Input: part model. Units: mm. Frame: model coordinates. Face numbers are marked on the shaded views. Coordinates: 2 decimals unless noted, no trailing zeros. Loops run counter-clockwise (first coordinate to the right, second up) from the corner with the lowest first, then second, coordinate; pieces in that order, holes last.
```python
from build123d import *

# Parameters (mm, degrees)
BOSS_EXTRUDE1_DEPTH           = 6.35
F_1_1_4_12_TAPPED_HOLE1_D     = 29.76626
F_1_1_4_12_TAPPED_HOLE1_DEPTH = 74.0791
F_1_1_4_12_TAPPED_HOLE1_TIP   = 8.942686705


with BuildPart() as part:
    # Sketch1 → Boss-Extrude1 (new body)
    with BuildSketch(Plane.XY):
        with BuildLine():
            Line((0, 0), (-25.4, 0))
            Line((-25.4, 0), (-25.4, 6.35))
            Line((-25.4, 6.35), (-18.344682017, 31.55167344))
            ThreePointArc((-18.344682017, 31.55167344), (0, 45.466), (18.344682017, 31.55167344))
            Line((18.344682017, 31.55167344), (25.4, 6.35))
            Line((25.4, 6.35), (25.4, 0))
            Line((25.4, 0), (0, 0))
        make_face()
    extrude(amount=BOSS_EXTRUDE1_DEPTH)

    # 1-1/4-12 Tapped Hole1
    with Locations(Plane(origin=(0, 26.416, 6.35), x_dir=(1, 0, 0), z_dir=(0, 0, 1))):
        with Locations((0, 0)):
            Hole(F_1_1_4_12_TAPPED_HOLE1_D / 2, depth=F_1_1_4_12_TAPPED_HOLE1_DEPTH)
            with Locations((0, 0, -(F_1_1_4_12_TAPPED_HOLE1_DEPTH + F_1_1_4_12_TAPPED_HOLE1_TIP / 2))):  # 118° drill point
                Cone(0, F_1_1_4_12_TAPPED_HOLE1_D / 2, F_1_1_4_12_TAPPED_HOLE1_TIP, mode=Mode.SUBTRACT)


solid = part.part
```
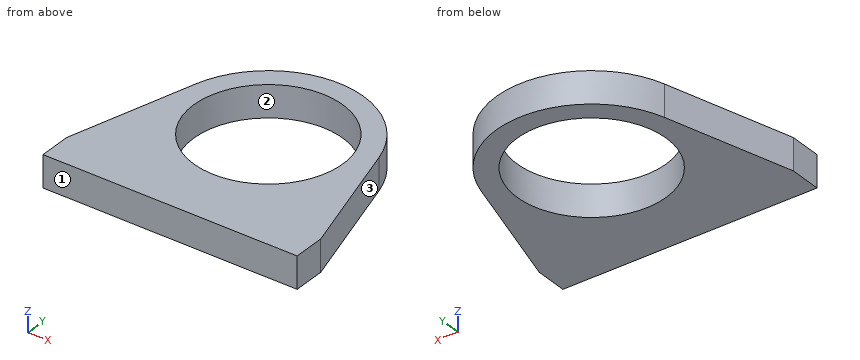
Item 1: Section query D-D (x = 17). Output: boundary loops of the cut face in (y, z).
Result:
outline: (0, 0) - (35.01, 0) - (35.01, 6.35) - (0, 6.35) - close
Item 2: Line query: L1, parallel to Y at x = 0, z = 4.5; L2, parallel to Y at x = -12, z = 1; L3, parallel to X at y = 31, z = 6. Output: solid intervals per line, ascending.
Result:
L1: y = 0 to 11.53, 41.3 to 45.47
L2: y = 0 to 17.61, 35.22 to 41.21
L3: x = -18.5 to -14.16, 14.16 to 18.5
Item 3: Section query A-A (x = 0). Output: boundary loops of the cut face in (y, z).
Result:
outline: (0, 0) - (11.53, 0) - (11.53, 6.35) - (0, 6.35) - close; (41.3, 0) - (45.47, 0) - (45.47, 6.35) - (41.3, 6.35) - close
Item 4: Section query C-C (z = 3). Output: boundary loops of the cut face in (x, y).
Result:
outline: (-25.4, 0) - (25.4, 0) - (25.4, 6.35) - (18.34, 31.55) arc R19.05 ccw to (-18.34, 31.55) - (-25.4, 6.35) - close; hole circle Ø29.77 at (0, 26.42)
Item 5: Section query B-B (y = 38.5). Output: boundary loops of the cut face in (x, z).
Result:
outline: (-14.73, 0) - (-8.69, 0) - (-8.69, 6.35) - (-14.73, 6.35) - close; (8.69, 0) - (14.73, 0) - (14.73, 6.35) - (8.69, 6.35) - close
Item 6: Contact query for flat-ended pins moving along their axis: P1, Ø1, axis at y = 25, z = 5.5, coming from the +X side; P2, Ø6, axis at x = 12.5, y = 4.5, coming from the -Z side; P3, Ø1.5, axis at y = 30.5, z = 2, coming from the -X side. Output: stop coordinate, or through.
Result:
P1: stops at x = 20.32
P2: stops at z = 0
P3: stops at x = -18.85
Item 7: Mould query, pull axis Y, two halves, no side actions, for the marked faces 1, 2 and 3. Classes: +Y half, -Y half, draft (parallel to the pull), parting line (faces both ways), or undercut.
Result:
face 1: -Y half
face 2: undercut
face 3: +Y half
